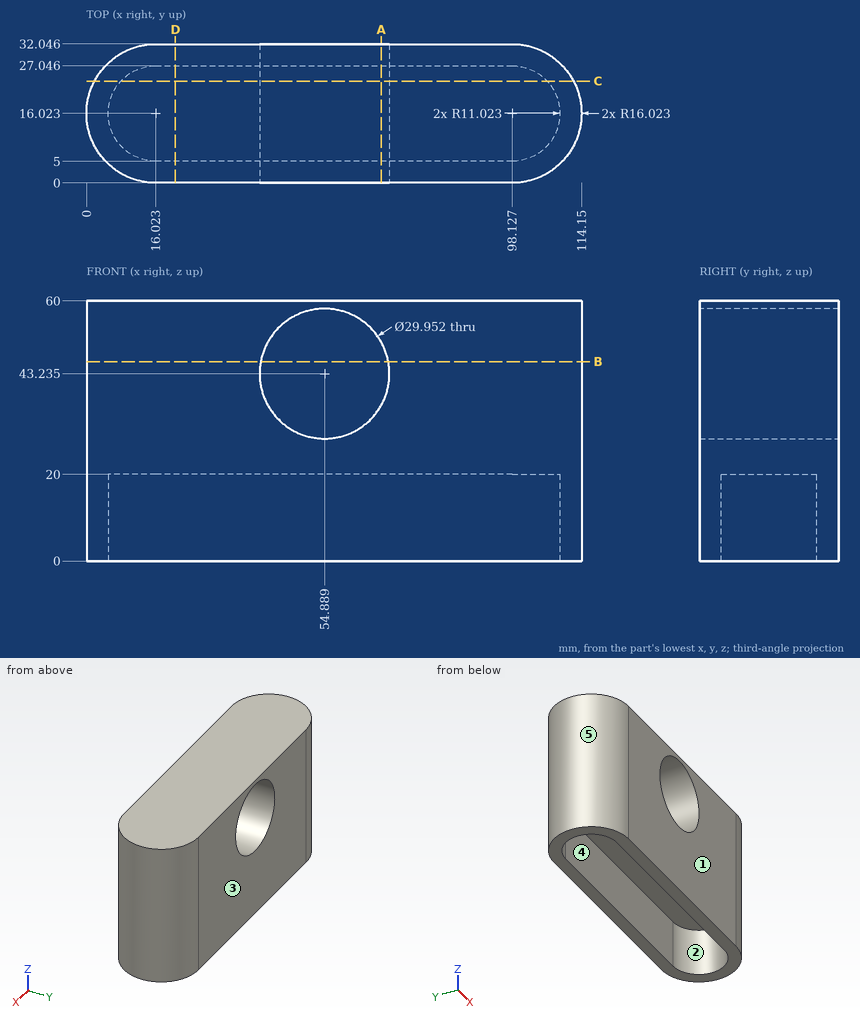
For this review, use the dimensioned drawing (mm, ordinates from the lowest corner) and the shaded views. A direction names the side the tool comes from. Coordinates: 2 decimals unless noted, no trailing zeros. Loops run counter-clockwise (first coordinate to the right, second up) from the corner with the lowest first, then second, coordinate; pieces in that order, holes last. Notation, with made-up numbers: (62, -13.75) - (105, -13.75) arc R11 ccw to (105, 6.25) - close; hole circle Ø7 at (31.5, 46). An arc over 180 degrees is marked (long way). Use one line per item in the form item = value. Start each with the question number.
1) Take a section at A-A (x = 68). State the section outline as (y, z) points.
2) For pin 1 (1.5 mm diameter, centred on y = 7, z = 49.5, fed in from +X); pin 2 (1 mm diameter, centred on x = 87.5, y = 22.5, fed in from -Z); pin 3 (5 mm diameter, centred on y = 24, z = 43.5, fed in from +X) (1 decimal), all flat-tipped, find the tip position at first contact; note any pin that passes through.
3) Take a section at B-B (z = 46). State the section outline as (x, y) points.
4) Draft analysis for pull direction Y (two halves, no side actions). For the marked faces 1, 2 and 3, state which applies: released by +Y, released by -Y, zero draft, split by the parting line, or undercut.
5) Take a section at D-D (x = 20.5). State the section outline as (y, z) points, plus the area to 3 significant figures.
6) Take a section at C-C (y = 23.5). State the section outline as (x, z) points (1 decimal), plus the area to 3 significant figures.
7) To check wall thickness, follow probe 1 along Z at (x, y) = (32, 18.5); probe 2 along X at (y, z) = (19.5, 32) (1 decimal); probe 3 along X at (y, z) = (16.5, 31) (1 decimal). State the ranges of each line that lie inside material, in increasing order. Write a range as from..to.
8) For the marked faces 4 and 5, list the 3-axis set-ups (+Z, -Z, +X, -X, +Y, -Y) from which the entire face can be reached by the end or side of a thin tool; tool diameter is ignored.
From the geometry:
q1.outline = (0, 0) - (5, 0) - (5, 20) - (27.05, 20) - (27.05, 0) - (32.05, 0) - (32.05, 36) - (0, 36) - close; (0, 50.47) - (32.05, 50.47) - (32.05, 60) - (0, 60) - close
q2.pin_1 = 111.85
q2.pin_2 = 20
q2.pin_3 = 113.2
q3.outline = (16.02, 0) - (40.17, 0) - (40.17, 32.05) - (16.02, 32.05) arc R16.02 ccw to start; (69.61, 0) - (98.13, 0) arc R16.02 ccw to (98.13, 32.05) - (69.61, 32.05) - close
q4.face_1 = released by -Y
q4.face_2 = undercut
q4.face_3 = released by +Y
q5.outline = (0, 0) - (5, 0) - (5, 20) - (27.05, 20) - (27.05, 0) - (32.05, 0) - (32.05, 60) - (0, 60) - close
q5.area = 1,480 mm2
q6.outline = (1.9, 0) - (7.9, 0) - (7.9, 20) - (106.2, 20) - (106.2, 0) - (112.3, 0) - (112.3, 60) - (1.9, 60) - close; hole circle Ø30 at (54.9, 43.2)
q6.area = 3,960 mm2
q7.probe_1 = 20..60
q7.probe_2 = 0.4..45, 64.8..113.8
q7.probe_3 = 0..46.3, 63.5..114.1
q8.face_4 = -Z
q8.face_5 = +Z, -Z, -X
